Work out the finished part from the listing and answer in its coordinate system (mm). Round coordinates to 2 decimals unless told otherwise and drop trailing zeros. Loops run counter-clockwise (first coordinate to the right, second up) from the corner with the lowest first, then second, coordinate; pieces in that order, holes last. Notation, with made-up numbers: (17, -36) - (27, -36) arc R30 cw to (27, -12) - close; hole circle Ø10 at (-35.5, 33). An arc over 180 degrees is marked (long way). Return JSON: item names as keys, results as strings.
from build123d import *

# Parameters (mm, degrees)
SKETCH_1_R      = 20
SKETCH_1_R_2    = 2.55
SKETCH_1_R_3    = 2.75
EXTRUDE_2_DEPTH = 4
FILLET_1_R      = 3


with BuildPart() as part:
    # Эскиз1 → Бобышка-Вытянуть2 (new body)
    with BuildSketch(Plane.XY):
        Polygon((-39.880822459, 0), (0, 39.880822459), (39.880822459, 0), (39.880822459, -50), (-39.880822459, -50), align=None)
        Circle(SKETCH_1_R, mode=Mode.SUBTRACT)
        with Locations((-33.333013665, 0)):
            Circle(SKETCH_1_R_2, mode=Mode.SUBTRACT)
        with Locations((0, 33.333013665)):
            Circle(SKETCH_1_R_2, mode=Mode.SUBTRACT)
        with Locations((33.333013665, 0)):
            Circle(SKETCH_1_R_2, mode=Mode.SUBTRACT)
        with Locations((-33, -44)):
            Circle(SKETCH_1_R_3, mode=Mode.SUBTRACT)
        with Locations((0, -44)):
            Circle(SKETCH_1_R_3, mode=Mode.SUBTRACT)
        with Locations((33, -44)):
            Circle(SKETCH_1_R_3, mode=Mode.SUBTRACT)
    extrude(amount=EXTRUDE_2_DEPTH)

    # Скругление1
    fillet_1_edges = [part.edges().sort_by_distance(p)[0] for p in [
        (-39.880822459, 0, 2),
        (0, 39.880822459, 2),
        (39.880822459, 0, 2),
        (39.880822459, -50, 2),
        (-39.880822459, -50, 2),
    ]]
    fillet(fillet_1_edges, radius=FILLET_1_R)


solid = part.part
1) Find the intervals of material crossed by L1, parallel to Y at x = 0, z = 1.8; L2, parallel to Y at x = 31.5, z = 1.65; L3, parallel to Y at x = -35, z = 1.15, in increasing order.
Verdict:
{"L1": "y = -50 to -46.75, -41.25 to -20, 20 to 30.78, 35.88 to 38.64", "L2": "y = -50 to -46.3, -41.7 to -1.77, 1.77 to 8.38", "L3": "y = -50 to -45.89, -42.11 to -1.93, 1.93 to 4.88"}
2) Determine the mould class of faces 1 (the flat face through (1, -50, 2)), 2 (the cylindrical face through (-0.358, -41.273, 1.972)), 3 (the cylindrical face through (39.646, -0.079, 2.028)) for opening direction X: pulls with the +X half, pulls with the -X half, needs draft (parallel to the pull), parting line crosses it, or undercut.
Verdict:
{"face 1": "needs draft", "face 2": "undercut", "face 3": "pulls with the +X half"}
3) Flat-ended cylindrical pins translate along their axes: pin 1 (4 mm diameter, centred on x = 0, y = 33.33, fed in from -Z); pin 2 (1 mm diameter, centred on x = 16, z = 2.5, fed in from +Y). Find the tip coordinate at first contact, or state that the pin passes through.
Verdict:
{"pin 1": "passes through", "pin 2": "stops at y = 24.38"}
4) Section B-B (x = 0) is taken. Give the vertices of the cut face in (y, z), and give its area (3 significant figures).
Verdict:
{"outline": "(-50, 0) - (-46.75, 0) - (-46.75, 4) - (-50, 4) - close; (-41.25, 0) - (-20, 0) - (-20, 4) - (-41.25, 4) - close; (20, 0) - (30.78, 0) - (30.78, 4) - (20, 4) - close; (35.88, 0) - (38.64, 0) - (38.64, 4) - (35.88, 4) - close", "area": "152 mm2"}
5) Section A-A (y = -12) is taken. Give the vertices of the cut face in (x, z), and give its area (3 significant figures).
Verdict:
{"outline": "(-39.88, 0) - (-16, 0) - (-16, 4) - (-39.88, 4) - close; (16, 0) - (39.88, 0) - (39.88, 4) - (16, 4) - close", "area": "191 mm2"}
6) Section C-C (y = -44) is taken. Give the vertices of the cut face in (x, z).
Verdict:
{"outline": "(-39.88, 0) - (-35.75, 0) - (-35.75, 4) - (-39.88, 4) - close; (-30.25, 0) - (-2.75, 0) - (-2.75, 4) - (-30.25, 4) - close; (2.75, 0) - (30.25, 0) - (30.25, 4) - (2.75, 4) - close; (35.75, 0) - (39.88, 0) - (39.88, 4) - (35.75, 4) - close"}
7) Section D-D (x = 33) is taken. Give the vertices of the cut face in (y, z).
Verdict:
{"outline": "(-50, 0) - (-46.75, 0) - (-46.75, 4) - (-50, 4) - close; (-41.25, 0) - (-2.53, 0) - (-2.53, 4) - (-41.25, 4) - close; (2.53, 0) - (6.88, 0) - (6.88, 4) - (2.53, 4) - close"}
